from build123d import *

# Parameters (mm, degrees)
SKETCH1_W                      = 32
SKETCH1_H                      = 55
BASE_FLANGE1_DEPTH             = 3
EDGE_FLANGE1_STRIP_W           = 13.4732
EDGE_FLANGE1_STRIP_H           = 3
EDGE_FLANGE1_STRIP_CUT_DEPTH   = 55
EDGE_FLANGE1_STRIP_2_W         = 13.4732
EDGE_FLANGE1_STRIP_2_H         = 3
EDGE_FLANGE1_STRIP_CUT_2_DEPTH = 55
EDGE_FLANGE1_DEPTH             = 55
EDGE_FLANGE1_BEND_DEPTH        = 55
CUT_EXTRUDE1_DEPTH             = 70.123078635
CUT_EXTRUDE2_DEPTH             = 70.123078635


# Sheet-metal steps are written as plain solids
with BuildPart() as part:
    # Sketch1 → Base-Flange1 (new body)
    with BuildSketch(Plane.XY):
        with Locations((16, 27.5)):
            Rectangle(SKETCH1_W, SKETCH1_H)
    extrude(amount=-BASE_FLANGE1_DEPTH)

    # Edge-Flange1 strip (across the edge) → Edge-Flange1 strip cut (cut)
    with BuildSketch(Plane(origin=(32, 0, 0), x_dir=(-1, 0, 0), z_dir=(0, 1, 0))):
        with Locations((-3, -1.5)):
            Rectangle(EDGE_FLANGE1_STRIP_W, EDGE_FLANGE1_STRIP_H)
    extrude(amount=EDGE_FLANGE1_STRIP_CUT_DEPTH, mode=Mode.SUBTRACT)

    # Edge-Flange1 strip 2 (across the edge) → Edge-Flange1 strip cut 2 (cut)
    with BuildSketch(Plane.XZ.offset(-55)):
        with Locations((-3, -1.5)):
            Rectangle(EDGE_FLANGE1_STRIP_2_W, EDGE_FLANGE1_STRIP_2_H)
    extrude(amount=EDGE_FLANGE1_STRIP_CUT_2_DEPTH, mode=Mode.SUBTRACT)

    # Edge-Flange1 section (across the edge) → Edge-Flange1 (add)
    with BuildSketch(Plane(origin=(32, 0, 0), x_dir=(-1, 0, 0), z_dir=(0, 1, 0))):
        with BuildLine():
            Line((0, 0.7366), (0, 27))
            Line((0, 27), (3, 27))
            Line((3, 27), (3, 0.7366))
            ThreePointArc((3, 0.7366), (3.215745145, 0.215745145), (3.7366, 0))
            Line((3.7366, 0), (3.7366, -3))
            ThreePointArc((3.7366, -3), (1.094424801, -1.905575199), (0, 0.7366))
        make_face()
    extrude(amount=EDGE_FLANGE1_DEPTH)

    # Edge-Flange1 section 2 (across the edge) → Edge-Flange1 bend (add)
    with BuildSketch(Plane.XZ.offset(-55)):
        with BuildLine():
            Line((0, 0.7366), (0, 27))
            Line((0, 27), (3, 27))
            Line((3, 27), (3, 0.7366))
            ThreePointArc((3, 0.7366), (3.215745145, 0.215745145), (3.7366, 0))
            Line((3.7366, 0), (3.7366, -3))
            ThreePointArc((3.7366, -3), (1.094424801, -1.905575199), (0, 0.7366))
        make_face()
    extrude(amount=EDGE_FLANGE1_BEND_DEPTH)

    # Sketch12 → Cut-Extrude1 (cut, through all)
    with BuildSketch(Plane.XY):
        with BuildLine():
            Line((13.5, 40.5), (18.5, 40.5))
            ThreePointArc((18.5, 40.5), (21.5, 37.5), (18.5, 34.5))
            Line((18.5, 34.5), (13.5, 34.5))
            ThreePointArc((13.5, 34.5), (10.5, 37.5), (13.5, 40.5))
        make_face()
        with BuildLine():
            Line((13.5, 20.5), (18.5, 20.5))
            ThreePointArc((18.5, 20.5), (21.5, 17.5), (18.5, 14.5))
            Line((18.5, 14.5), (13.5, 14.5))
            ThreePointArc((13.5, 14.5), (10.5, 17.5), (13.5, 20.5))
        make_face()
    extrude(amount=-CUT_EXTRUDE1_DEPTH, mode=Mode.SUBTRACT)

    # Sketch13 → Cut-Extrude2 (cut, through all)
    with BuildSketch(Plane(origin=(32, 0, 0), x_dir=(0, 0, -1), z_dir=(1, 0, 0))):
        with BuildLine():
            Line((-12, 55), (-12, 47))
            ThreePointArc((-12, 47), (-15, 44), (-18, 47))
            Line((-18, 47), (-18, 55))
            ThreePointArc((-18, 55), (-15, 58), (-12, 55))
        make_face()
        with BuildLine():
            Line((-12, 25), (-12, 9))
            ThreePointArc((-12, 9), (-15, 6), (-18, 9))
            Line((-18, 9), (-18, 25))
            ThreePointArc((-18, 25), (-15, 28), (-12, 25))
        make_face()
    extrude(amount=-CUT_EXTRUDE2_DEPTH, mode=Mode.SUBTRACT)


solid = part.part
Work out the finished part from the listing and answer in its coordinate system (mm). A direction names the side the tool comes from. Round coordinates to 2 decimals unless told otherwise and drop trailing zeros. Loops run counter-clockwise (first coordinate to the right, second up) from the corner with the lowest first, then second, coordinate; pieces in that order, holes last. Notation, with made-up numbers: (22, -9) - (42, -9) arc R31 ccw to (42, 23) - close; hole circle Ø1 at (78.25, 85). An arc over 180 degrees is marked (long way). Use one line per item in the form item = value. Start each with the question number.
(1) Find section B-B on y = 17.5. Determine the outline of the cut face in (x, z), and give its area (3 significant figures).
(2) Determine the mould class of faces 5 (the face through (16, 34.5, -1)), 6 (the face through (2, 28, 15)), 7 (the face through (30.88, 27.12, -1.93)) for opening direction X: +X half, -X half, draft (parallel to the pull), parting line (faces both ways), or undercut.
(3) Find section C-C on x = 14.5. Determine the outline of the cut face in (y, z), and give its area (3 significant figures).
(4) Find section D-D on y = 12. Determine the outline of the cut face in (x, z).
(5) Consider line 1 (X direction, y = 40.5, z = 2.25); line 2 (Z direction, x = 18.5, y = 48). Determine where each line is inside the solid, lowest interval first.
(6) Find section A-A on z = 18.75. Determine the outline of the cut face in (x, y), and give its area (3 significant figures).
(7) Which of the six approach directions +Z, -Z, +X, -X, +Y, -Y give full straight-line access (tool end or side, diameter ignored) to faces 1 (the face through (31, 51, 18)), 2 (the face through (31, 28, 15)), 3 (the face through (10.5, 37.4, -1.5)), 4 (the face through (16, 28, 0))?
(8) Flat-ended cylindrical pins translate along their axes: P1, Ø0.9, axis at x = 1, y = 13.5, coming from the -Z side; P2, Ø8, axis at x = 10.5, z = 8.5, coming from the -Y side; P3, Ø1, axis at x = 8, y = 7.5, coming from the +Z side; P4, Ø0.9, axis at x = 30, y = 49.5, coming from the -Z side. Find the tip coordinate at first contact, or state that the pin passes through.
Answer list:
q1.outline = (0, 0.74) arc R3.74 ccw to (3.74, -3) - (10.5, -3) - (10.5, 0) - (3.74, 0) arc R0.74 cw to (3, 0.74) - (3, 12) - (0, 12) - close; (0, 18) - (3, 18) - (3, 27) - (0, 27) - close; (21.5, -3) - (28.26, -3) arc R3.74 ccw to (32, 0.74) - (32, 12) - (29, 12) - (29, 0.74) arc R0.74 cw to (28.26, 0) - (21.5, 0) - close; (29, 18) - (32, 18) - (32, 27) - (29, 27) - close
q1.area = 183 mm^2
q2.face_5 = undercut
q2.face_6 = draft
q2.face_7 = +X half
q3.outline = (0, -3) - (14.5, -3) - (14.5, 0) - (0, 0) - close; (20.5, -3) - (34.5, -3) - (34.5, 0) - (20.5, 0) - close; (40.5, -3) - (55, -3) - (55, 0) - (40.5, 0) - close
q3.area = 129 mm^2
q4.outline = (0, 0.74) arc R3.74 ccw to (3.74, -3) - (28.26, -3) arc R3.74 ccw to (32, 0.74) - (32, 12) - (29, 12) - (29, 0.74) arc R0.74 cw to (28.26, 0) - (3.74, 0) arc R0.74 cw to (3, 0.74) - (3, 12) - (0, 12) - close; (0, 18) - (3, 18) - (3, 27) - (0, 27) - close; (29, 18) - (32, 18) - (32, 27) - (29, 27) - close
q5.line_1 = 0 to 3, 29 to 32
q5.line_2 = -3 to 0
q6.outline = (0, 0) - (3, 0) - (3, 55) - (0, 55) - close; (29, 0) - (32, 0) - (32, 55) - (29, 55) - close
q6.area = 330 mm^2
q7.face_1 = +X, -X, +Y
q7.face_2 = +X, -X
q7.face_3 = +Z, -Z
q7.face_4 = +Z, +Y, -Y
q8.P1 = -2.22
q8.P2 = through
q8.P3 = 0
q8.P4 = -2.77
